```python
from build123d import *

# Parameters (mm, degrees)
CROQUIS1_W              = 12
CROQUIS1_H              = 3
SALIENTE_EXTRUIR1_DEPTH = 3
CROQUIS2_W              = 3
CROQUIS2_H              = 3
SALIENTE_EXTRUIR2_DEPTH = 3


with BuildPart() as part:
    # Croquis1 → Saliente-Extruir1 (new body)
    with BuildSketch(Plane.XY):
        Polygon((0, 0), (3, 0), (3, 3), (15, 3), (15, 0), (85, 0), (85, 3), (97, 3), (97, 0), (100, 0), (100, 29), (0, 29), align=None)
        with Locations((9, 21.5)):
            Rectangle(CROQUIS1_W, CROQUIS1_H, mode=Mode.SUBTRACT)
        with Locations((91, 21.5)):
            Rectangle(CROQUIS1_W, CROQUIS1_H, mode=Mode.SUBTRACT)
    extrude(amount=SALIENTE_EXTRUIR1_DEPTH)

    # Croquis2 → Saliente-Extruir2 (add)
    with BuildSketch(Plane.XY.offset(3)):
        with Locations((-1.5, 21.5)):
            Rectangle(CROQUIS2_W, CROQUIS2_H)
        with Locations((-1.5, 27.5)):
            Rectangle(CROQUIS2_W, CROQUIS2_H)
    extrude(amount=-SALIENTE_EXTRUIR2_DEPTH)


solid = part.part
```
CAD build for the part. Positions are in the model's coordinates, mm. A direction names the side the tool comes from. Coordinates: 2 decimals unless noted, no trailing zeros. Write each loop counter-clockwise with the first axis right and the second up, starting at its lowest first coordinate (ties: lowest second). Pieces come first, ordered by that corner, then holes. Notation, with made-up numbers: (64, 56.5) -> (96, 56.5) arc R18 ccw to (96, 69.5) -> close; hole circle Ø8 at (26.25, 49.5). An arc over 180 degrees is marked (long way). Return JSON: item names as keys, results as strings. Group by question number.
Q1. Which spindle directions (+Z, -Z, +X, -X, +Y, -Y) get a long thin tool onto all of the face, cutting with end or side? Do faces 5 (the face through (9, 3, 1)), 6 (the face through (-2, 23, 2)), 7 (the face through (9, 23, 1)), 8 (the face through (-2, 20, 2)). Say none if no direction does.
Q2. Cut at B-B, the plane y = 21. Give the cut face in (x, z), then the cut area to 3 significant figures.
Q3. Pull direction X, two halves, no side cores. Call faces 1 (the face through (-2, 26, 2)), 2 (the face through (91, 3, 1)), 3 (the face through (97, 21, 1)), 4 (the face through (-3, 21, 2)): released by +X, released by -X, zero draft, split by the parting line, or undercut.
Q4. Drill centre lines: line 1 (X direction, y = 21.75, z = 0.5); line 2 (X direction, y = 2.75, z = 2.4); line 3 (Y direction, x = 92, z = 0.95). Where is each one in solid material? Low to high.
Q5. Cut at C-C, the plane x = 94. Give the cut face in (y, z), then the cut area to 3 significant figures.
Q6. Cut at D-D, the plane y = 4. Give the cut face in (x, z), then the cut area to 3 significant figures.
Q7. Cut at A-A, the plane z = 1.3. Give the cut face in (x, y).
Q8. Flat gauge pins, fed straight in: pin 1 (4 mm diameter, centred on x = 37.5, y = 23, fed in from -Z); pin 2 (1.5 mm diameter, centred on y = 9, z = 1, fed in from -X). Where does each tip first touch, or does it go through?
Returned:
{
 "1": {"face 5": "+Z, -Z, -Y", "face 6": "+Z, -Z, -X", "face 7": "+Z, -Z", "face 8": "+Z, -Z, -X, -Y"},
 "2": {"outline": "(-3, 0) -> (3, 0) -> (3, 3) -> (-3, 3) -> close; (15, 0) -> (85, 0) -> (85, 3) -> (15, 3) -> close; (97, 0) -> (100, 0) -> (100, 3) -> (97, 3) -> close", "area": "237 mm2"},
 "3": {"face 1": "zero draft", "face 2": "undercut", "face 3": "undercut", "face 4": "released by -X"},
 "4": {"line 1": "x = -3 to 3, 15 to 85, 97 to 100", "line 2": "x = 0 to 3, 15 to 85, 97 to 100", "line 3": "y = 3 to 20, 23 to 29"},
 "5": {"outline": "(3, 0) -> (20, 0) -> (20, 3) -> (3, 3) -> close; (23, 0) -> (29, 0) -> (29, 3) -> (23, 3) -> close", "area": "69.0 mm2"},
 "6": {"outline": "(0, 0) -> (100, 0) -> (100, 3) -> (0, 3) -> close", "area": "300 mm2"},
 "7": {"outline": "(-3, 20) -> (0, 20) -> (0, 0) -> (3, 0) -> (3, 3) -> (15, 3) -> (15, 0) -> (85, 0) -> (85, 3) -> (97, 3) -> (97, 0) -> (100, 0) -> (100, 29) -> (-3, 29) -> (-3, 26) -> (0, 26) -> (0, 23) -> (-3, 23) -> close; hole (3, 20) -> (15, 20) -> (15, 23) -> (3, 23) -> close; hole (85, 20) -> (97, 20) -> (97, 23) -> (85, 23) -> close"},
 "8": {"pin 1": "stops at z = 0", "pin 2": "stops at x = 0"}
}
